Part model, mm, in its own coordinate system. A direction names the side the tool comes from. Round coordinates to 2 decimals unless told otherwise and drop trailing zeros. Loops run counter-clockwise (first coordinate to the right, second up) from the corner with the lowest first, then second, coordinate; pieces in that order, holes last.
(1) Tool access for faces 1 (the face through (1422.364, 69, 17)), 2 (the face through (1423.951, 69, 13)): list every direction of +Z, -Z, +X, -X, +Y, -Y with a clear straight run to the whole face (end or side of a thin tool).
(2) Flat gauge pins, fed straight in: pin 1 (6 mm diameter, centred on x = 310.5, y = 134, fed in from -Z); pin 2 (1.7 mm diameter, centred on x = 1423.5, z = 16, fed in from -Y); pin 3 (1.7 mm diameter, centred on x = 1423, z = 17.5, fed in from +Y). Where does each tip first touch, or does it go through?
(3) Cut at B-B on x = 1013.5. List the corners of the cut face in (y, z), then the cut area to 3 significant figures.
(4) Probe probe 1 along Z at (x, y) = (439, 58.5); probe 2 along X at (y, z) = (68.5, 17). List the from-to ranges inside material, lowest first.
(5) Cut at A-A on z = 16. List the corners of the cut face in (x, y), then the cut area to 3 significant figures.
(6) Cut at C-C on y = 22. List the corners of the cut face in (x, z), then the cut area to 3 significant figures.
from build123d import *

# Parameters (mm, degrees)
F0_W     = 1500
F0_H     = 178
F1_DEPTH = 1.5875
F2_W     = 30
F2_H     = 30
F3_DEPTH = 1.5875


# Not quite as in the source:
# - a length typed as a fraction of an inch, garbled in the dataset ("3 / 203.2 mm" for 3/8 in), is restored


with BuildPart() as f1:
    # F0 (on Top) → F1 (new body)
    with BuildSketch(Plane.XY):
        with Locations((673.9510029554, 75.5837445271)):
            Rectangle(F0_W, F0_H)
    extrude(amount=F1_DEPTH)

    # F2 (on face) → F3 (join)
    with BuildSketch(Plane.YZ.offset(1423.9510029554)):
        with Locations((75.5837445271, 16.5875)):
            Rectangle(F2_W, F2_H)
        with BuildLine():
            ThreePointArc((71.5837445271, 24.0875), (75.5837445271, 28.0875), (79.5837445271, 24.0875))
            Line((79.5837445271, 24.0875), (79.5837445271, 9.0875))
            ThreePointArc((79.5837445271, 9.0875), (75.5837445271, 5.0875), (71.5837445271, 9.0875))
            Line((71.5837445271, 9.0875), (71.5837445271, 24.0875))
        make_face(mode=Mode.SUBTRACT)
    extrude(amount=-F3_DEPTH)


solid = f1.part
Final values:
1. face 1: +Z, -X, +Y, -Y
1. face 2: +Z, -Z, +X, +Y, -Y
2. pin 1: stops at z = 0
2. pin 2: stops at y = 60.58
2. pin 3: stops at y = 90.58
3. outline: (-13.42, 0) - (164.58, 0) - (164.58, 1.59) - (-13.42, 1.59) - close
3. area: 283 mm2
4. probe 1: z = 0 to 1.59
4. probe 2: x = 1422.36 to 1423.95
5. outline: (1422.36, 60.58) - (1423.95, 60.58) - (1423.95, 71.58) - (1422.36, 71.58) - close; (1422.36, 79.58) - (1423.95, 79.58) - (1423.95, 90.58) - (1422.36, 90.58) - close
5. area: 34.9 mm2
6. outline: (-76.05, 0) - (1423.95, 0) - (1423.95, 1.59) - (-76.05, 1.59) - close
6. area: 2,380 mm2
